Input: dimensioned drawing with shaded views. Units: mm. Origin: part minimum x, y, z. A direction names the side the tool comes from. Round coordinates to 2 decimals unless told otherwise and drop trailing zeros. Loops run counter-clockwise (first coordinate to the right, second up) from the corner with the lowest first, then second, coordinate; pieces in that order, holes last. Notation, with made-up numbers: (-23.5, 35) - (-11.5, 35) arc R25 ccw to (-11.5, 65) - close; hole circle Ø1 at (-20.75, 70.25). An arc over 180 degrees is marked (long way). Write each question's results on one line, items separated by ' | '.
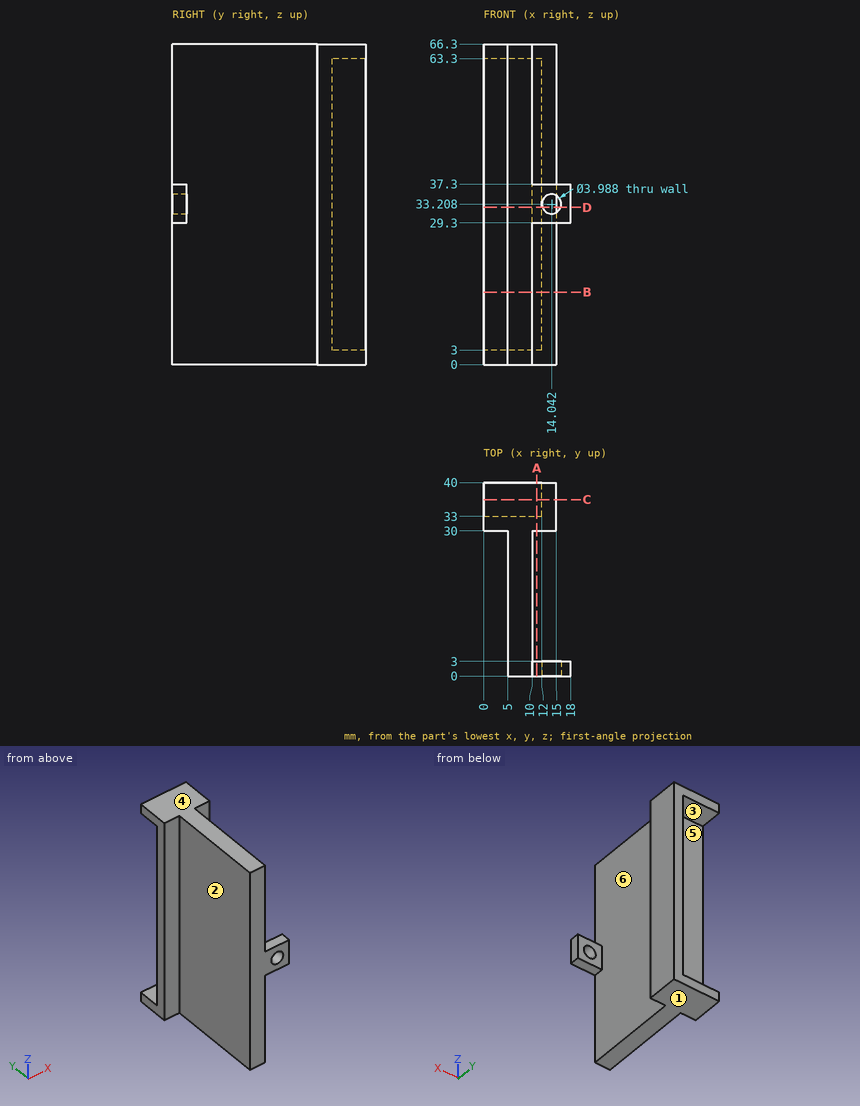
1. Section query D-D, the plane z = 32.5. Output: boundary loops of the cut face in (x, y), plus the area to 3 significant figures.
Answer:
outline: (0, 30) - (5, 30) - (5, 0) - (12.18, 0) - (12.18, 3) - (10, 3) - (10, 30) - (15, 30) - (15, 40) - (12, 40) - (12, 33) - (0, 33) - close; (15.91, 0) - (18, 0) - (18, 3) - (15.91, 3) - close | area: 229 mm^2
2. Section query A-A, the plane x = 11. Output: boundary loops of the cut face in (y, z).
Answer:
outline: (0, 29.3) - (3, 29.3) - (3, 37.3) - (0, 37.3) - close; (30, 0) - (40, 0) - (40, 3) - (33, 3) - (33, 63.3) - (40, 63.3) - (40, 66.3) - (30, 66.3) - close
3. Mould query, pull axis Z, two halves, no side actions, for the marked faces 3, 4, 5 and 6. Classes: pulls with the +Z half, pulls with the -Z half, needs draft (parallel to the pull), parting line crosses it, or undercut.
Answer:
face 3: undercut | face 4: pulls with the +Z half | face 5: undercut | face 6: needs draft
4. Section query B-B, the plane z = 15. Output: boundary loops of the cut face in (x, y).
Answer:
outline: (0, 30) - (5, 30) - (5, 0) - (10, 0) - (10, 30) - (15, 30) - (15, 40) - (12, 40) - (12, 33) - (0, 33) - close
5. Section query C-C, the plane y = 36.5. Output: boundary loops of the cut face in (x, z).
Answer:
outline: (0, 0) - (15, 0) - (15, 66.3) - (0, 66.3) - (0, 63.3) - (12, 63.3) - (12, 3) - (0, 3) - close
6. Line query: line 1 (Z direction, x = 7.5, y = 37.5); line 2 (Y direction, x = 14.75, z = 8); line 3 (X direction, y = 11.5, z = 60). Output: solid intervals per line, ascending. Write a range as [from, to].
Answer:
line 1: [0, 3], [63.3, 66.3] | line 2: [30, 40] | line 3: [5, 10]
7. Set-up query: the marked faces 1 and 2. Return all of +Z, -Z, +X, -X, +Y, -Y with unobstructed straight access to the full face (end or side cutting, diameter ignored); none if empty.
Answer:
face 1: -Z, +X, -X, +Y, -Y | face 2: +Z, -Z, -X, -Y
8. Contact query for flat-ended pins moving along their axis: pin 1 (15 mm diameter, centred on y = 16, z = 40.5, fed in from +X); pin 2 (9.5 mm diameter, centred on x = 3.5, z = 23, fed in from +Y); pin 3 (2 mm diameter, centred on y = 37.5, z = 19.5, fed in from -X). Output: stop coordinate, or through.
Answer:
pin 1: x = 10 | pin 2: y = 33 | pin 3: x = 12
